```python
from build123d import *

# Parameters (mm, degrees)
SKETCH3_R          = 0.347265625
CUT_EXTRUDE1_DEPTH = 0.3175


with BuildPart() as part:
    # Sketch2 → Revolve1 (revolve)
    with BuildSketch(Plane.XY):
        with BuildLine():
            Line((0, 3.175), (0, -9.525))
            Line((0, -9.525), (3.224609375, -9.525))
            Line((3.224609375, -9.525), (4.9609375, -6.35))
            Line((4.9609375, -6.35), (3.20675, -6.35))
            ThreePointArc((3.20675, -6.35), (3.18429936, -6.34070064), (3.175, -6.31825))
            Line((3.175, -6.31825), (3.175, -0.03175))
            ThreePointArc((3.175, -0.03175), (3.18429936, -0.00929936), (3.20675, 0))
            Line((3.20675, 0), (6.35, 0))
            Line((6.35, 0), (6.35, 2.8575))
            ThreePointArc((6.35, 2.8575), (6.257006403, 3.082006403), (6.0325, 3.175))
            Line((6.0325, 3.175), (0, 3.175))
        make_face()
    revolve(axis=Axis((0, 3.175, 0), (0, -1, 0)))

    # Sketch3 → Cut-Extrude1 (cut)
    with BuildSketch(Plane.XZ.offset(9.525)):
        with Locations((0, 2.28203125)):
            Circle(SKETCH3_R)
        with Locations((1.976297035, -1.141015625)):
            Circle(SKETCH3_R)
        with Locations((-1.976297035, -1.141015625)):
            Circle(SKETCH3_R)
    extrude(amount=-CUT_EXTRUDE1_DEPTH, mode=Mode.SUBTRACT)


solid = part.part
```
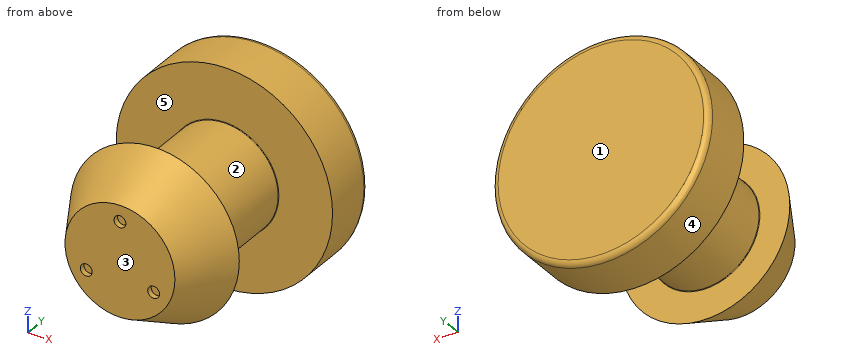
Here's how the part is built. I have some questions about the finished solid (model axes, mm). Face numbers are marked on the shaded views. A direction names the side the tool comes from. Give positions to 0.01 mm unless a question says otherwise; leave off trailing zeros. Write each loop counter-clockwise with the first axis right and the second up, starting at its lowest first coordinate (ties: lowest second). Pieces come first, ordered by that corner, then holes. Notation, with made-up numbers: M 38,30.5 L 72,30.5 A17 cw 72,44.5 Z; hole C 47.5,82.5 d1. An arc over 180 degrees is marked long. Put each result on its own line as item: value. Start each with the question number.
Item 1: Thinking about a two-plate mould opening in Y: for the marked faces 1, 2 and 3, which applies, +Y half, -Y half, draft (parallel to the pull), parting line (faces both ways), or undercut?
Item 2: If we section it at C-C, the plane y = -2.25: Write out the boundary of the cut face in (x, z) (3 decimals).
Item 3: On a 3-axis mill with a long thin cutter (end or side, diameter ignored), from which of +Z, -Z, +X, -X, +Y, -Y can I reach the whole of each face in a straight line? I mean the marked faces 4 and 5. Say none if no direction works.
Item 4: I need wall thicknesses on L1, parallel to Y at x = -0.5, z = 5.5 (3 decimals); L2, parallel to Z at x = 0, y = -9.35; L3, parallel to Y at x = -3.25, z = 2 (3 decimals). Which ranges of each line are inside material? Lowest first, please. Write a range as from..to.
Item 5: Will these pins go through, and if not, where does the flat tip stop? pin 1 (1.5 mm diameter, centred on y = -8, z = 1.5, fed in from -X); pin 2 (2 mm diameter, centred on y = -2, z = 4.5, fed in from -X); pin 3 (6 mm diameter, centred on y = -1, z = -4, fed in from -X).
Values:
1. face 1: +Y half
1. face 2: undercut
1. face 3: -Y half
2. outline: C 0,0 d6.35
3. face 4: +Y, -Y
3. face 5: none
4. L1: 0..3.175
4. L2: -3.32..1.93, 2.63..3.32
4. L3: -8.443..-6.35, 0..3.175
5. pin 1: x = -4.27
5. pin 2: through
5. pin 3: x = -6.24
